Part model, mm, in its own coordinate system. A direction names the side the tool comes from. Give positions to 0.01 mm unless a question says otherwise; leave off trailing zeros. Loops run counter-clockwise (first coordinate to the right, second up) from the corner with the lowest first, then second, coordinate; pieces in that order, holes last. Notation, with made-up numbers: (22.25, 21.25) -> (78.25, 21.25) arc R24 ccw to (78.25, 47.25) -> close; hole circle Ø11 at (7.5, -11). An arc over 180 degrees is marked (long way). Write item = value, one per line.
from build123d import *

# Parameters (mm, degrees)
SKETCH1_R                      = 8.7
BOSS_EXTRUDE1_DEPTH            = 15
SKETCH5_R                      = 1.75
CUT_EXTRUDE1_DEPTH             = 20.400515457
SKETCH6_R                      = 2.65
CUT_EXTRUDE3_DEPTH             = 6.4
SKETCH2_W                      = 17
SKETCH2_H                      = 4.566888769
CUT_EXTRUDE4_DEPTH             = 11
FILLET1_R                      = 0.3
TAP_DRILL_FOR_M2_5X0_45_TAP2_D = 2.05
SKETCH4_R                      = 2
BOSS_EXTRUDE2_DEPTH            = 3


with BuildPart() as part:
    # Sketch1 → Boss-Extrude1 (new body)
    with BuildSketch(Plane.XY):
        Circle(SKETCH1_R)
    extrude(amount=BOSS_EXTRUDE1_DEPTH)

    # Sketch5 → Cut-Extrude1 (cut, through all)
    with BuildSketch(Plane(origin=(0, 0, 0), x_dir=(-1, 0, 0), z_dir=(0, 0, -1))):
        Circle(SKETCH5_R)
    extrude(amount=-CUT_EXTRUDE1_DEPTH, mode=Mode.SUBTRACT)

    # Sketch6 → Cut-Extrude3 (cut)
    with BuildSketch(Plane.XY.offset(15)):
        Circle(SKETCH6_R)
    extrude(amount=-CUT_EXTRUDE3_DEPTH, mode=Mode.SUBTRACT)

    # Sketch2 → Cut-Extrude4 (cut)
    with BuildSketch(Plane.XY.offset(15)):
        with Locations((0.844453543, 6.416555616)):
            Rectangle(SKETCH2_W, SKETCH2_H)
    extrude(amount=-CUT_EXTRUDE4_DEPTH, mode=Mode.SUBTRACT)

    # Fillet1
    fillet1_edges = [part.edges().sort_by_distance(p)[0] for p in [
        (1.75, 0, 8.6),
    ]]
    fillet(fillet1_edges, radius=FILLET1_R)

    # Tap Drill for M2.5x0.45 Tap2 (through all)
    with Locations(Plane(origin=(0, 4.133111231, 0), x_dir=(1, 0, 0), z_dir=(0, 1, 0))):
        with Locations((-4.355546457, -9.5), (4.644453543, -9.5)):
            Hole(TAP_DRILL_FOR_M2_5X0_45_TAP2_D / 2)

    # Sketch4 → Boss-Extrude2 (add)
    with BuildSketch(Plane(origin=(0, 0, 0), x_dir=(-1, 0, 0), z_dir=(0, 0, -1))):
        with Locations(Location((0, 6, 0), (0, 0, 180))):
            Circle(SKETCH4_R)
        with Locations(Location((6, 0, 0), (0, 0, 180))):
            Circle(SKETCH4_R)
        with Locations(Location((0, -6, 0), (0, 0, 180))):
            Circle(SKETCH4_R)
        with Locations(Location((-6, 0, 0), (0, 0, 180))):
            Circle(SKETCH4_R)
    extrude(amount=BOSS_EXTRUDE2_DEPTH)


solid = part.part
1) Slice it at A-A, the plane y = 0. List the corners of the cut face in (x, z) (3 decimals), and give its area (3 significant figures).
Resolved:
outline = (-8.7, 0) -> (-8, 0) -> (-8, -3) -> (-4, -3) -> (-4, 0) -> (-1.75, 0) -> (-1.75, 8.3) arc R0.3 ccw to (-2.05, 8.6) -> (-2.65, 8.6) -> (-2.65, 15) -> (-8.7, 15) -> close; (1.75, 0) -> (4, 0) -> (4, -3) -> (8, -3) -> (8, 0) -> (8.7, 0) -> (8.7, 15) -> (2.65, 15) -> (2.65, 8.6) -> (2.05, 8.6) arc R0.3 ccw to (1.75, 8.3) -> close; hole circle Ø2.05 at (-4.356, 9.5); hole circle Ø2.05 at (4.644, 9.5)
area = 214 mm²
2) Drop flat-ended pins along their axis: P1, Ø3, axis at y = -4.5, z = 8, coming from the -X side; P2, Ø3.5, axis at x = -4.36, z = 9.5, coming from the +Y side; P3, Ø9, axis at x = -3, z = 7, coming from the +Y side; P4, Ø1, axis at y = 4, z = 8, coming from the -X side. Give the stop position or say it passes through.
Resolved:
P1 = -8.17
P2 = 4.13
P3 = 8.7
P4 = -7.96
3) Pull direction Y, two halves, no side cores. Call faces 5 (the face through (-1.886, -8.493, 7.395)), 6 (the face through (2.45, -1.01, 11.84)), 7 (the face through (-3.33, -2.04, 9.45)), 8 (the face through (0, 4.133, 10)): pulls with the +Y half, pulls with the -Y half, needs draft (parallel to the pull), parting line crosses it, or undercut.
Resolved:
face_5 = parting line crosses it
face_6 = undercut
face_7 = needs draft
face_8 = pulls with the +Y half
4) Slice it at C-C, the plane z = 10.25. List the corners of the cut face in (x, y), and give its area (3 significant figures).
Resolved:
outline = (-7.66, 4.13) arc R8.7 ccw to (-5.05, -7.08) -> (-5.05, 4.13) -> close; (-3.66, -7.89) arc R8.7 ccw to (3.95, -7.75) -> (3.95, 4.13) -> (-3.66, 4.13) -> close; (5.34, -6.87) arc R8.7 ccw to (7.66, 4.13) -> (5.34, 4.13) -> close; hole circle Ø5.3 at (0, 0)
area = 134 mm²
5) Which spindle directions (+Z, -Z, +X, -X, +Y, -Y) get a long thin tool onto all of the face, cutting with end or side? Do faces 1 (the face through (0, 6, 4)), 2 (the face through (0, 8, -1)), 3 (the face through (1, -2, 8.6)), 4 (the face through (6, 0, -3)). Say none if no direction does.
Resolved:
face_1 = +Z, +X, -X, +Y
face_2 = -Z
face_3 = +Z
face_4 = -Z, +X, -X, +Y, -Y
6) Drill centre lines: line 1 along X through (y, z) = (-3, 9.5); line 2 along X through (y, z) = (-1, 9); line 3 along Z through (x, y) = (4.75, 3.25). Where is each one in solid material? Low to high. Write a range as [from, to].
Resolved:
line_1 = [-8.17, -5.38], [-3.33, 3.62], [5.67, 8.17]
line_2 = [-8.64, -5.25], [-3.46, -2.45], [2.45, 3.75], [5.54, 8.64]
line_3 = [0, 8.48], [10.52, 15]
7) Slice it at B-B, the plane y = -6. List the corners of the cut face in (x, z) (3 decimals), and give its area (3 significant figures).
Resolved:
outline = (-6.3, 0) -> (-2, 0) -> (-2, -3) -> (2, -3) -> (2, 0) -> (6.3, 0) -> (6.3, 15) -> (-6.3, 15) -> close; hole circle Ø2.05 at (-4.356, 9.5); hole circle Ø2.05 at (4.644, 9.5)
area = 194 mm²
8) Slice it at D-D, the plane x = -6. List the corners of the cut face in (y, z).
Resolved:
outline = (-6.3, 0) -> (-2, 0) -> (-2, -3) -> (2, -3) -> (2, 0) -> (6.3, 0) -> (6.3, 4) -> (4.13, 4) -> (4.13, 15) -> (-6.3, 15) -> close
